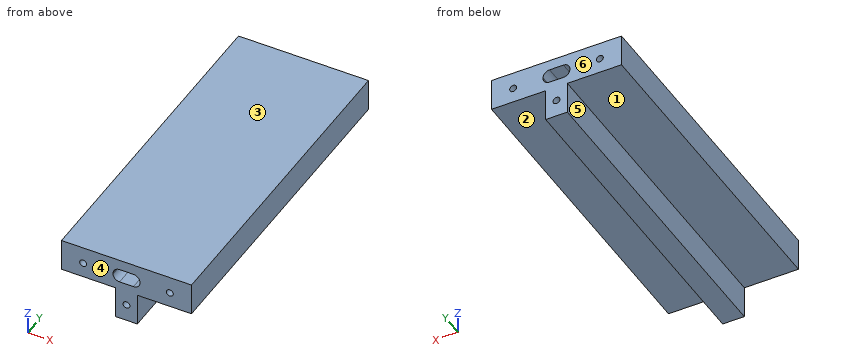
```python
from build123d import *

# Parameters (mm, degrees)
BOSS_EXTRUDE1_DEPTH        = 37.5
SKETCH2_W                  = 6.2
SKETCH2_H                  = 3.2
CUT_EXTRUDE1_DEPTH         = 6.2
FILLET1_R                  = 1.5
M2_TAPPED_HOLE1_AT_2_COUNT = 2
M2_TAPPED_HOLE1_AT_2_PITCH = 12.206555616
M2_TAPPED_HOLE1_AT_3_COUNT = 2
M2_TAPPED_HOLE1_AT_3_PITCH = 20
FILLET1_OF_MIRROR1_R       = 1.5


with BuildPart() as part:
    # Sketch1 → Boss-Extrude1 (new body, symmetric)
    with BuildSketch(Plane(origin=(0, 0, 0), x_dir=(1, 0, 0), z_dir=(0, 1, 0))):
        Polygon((-15, 0), (15, 0), (15, 7.5), (2.5, 7.5), (2.5, 15), (-2.5, 15), (-2.5, 7.5), (-15, 7.5), align=None)
    extrude(amount=BOSS_EXTRUDE1_DEPTH, both=True)

    # Sketch2 → Cut-Extrude1 (cut)
    with BuildSketch(Plane.XZ.offset(37.5)):
        with Locations((0, -4)):
            Rectangle(SKETCH2_W, SKETCH2_H)
    cut_extrude1 = extrude(amount=-CUT_EXTRUDE1_DEPTH, mode=Mode.SUBTRACT)

    # Fillet1
    fillet1_edges = [part.edges().sort_by_distance(p)[0] for p in [
        (-3.1, -34.4, -5.6),
        (-3.1, -34.4, -2.4),
        (3.1, -34.4, -2.4),
        (3.1, -34.4, -5.6),
    ]]
    fillet(fillet1_edges, radius=FILLET1_R)

    # Sketch6 → M2 Tapped Hole1 (revolve, cut)
    with BuildSketch(Plane(origin=(-10, -37.5, -4), x_dir=(0, 0, -1), z_dir=(1, 0, 0))):
        Polygon((0, 0), (0, 5.680688495), (0.8, 5.2), (0.8, 0), align=None)
    m2_tapped_hole1 = revolve(axis=Axis((-10, -43.85, -4), (0, 1, 0)), mode=Mode.SUBTRACT)

    # M2 Tapped Hole1 at 2: M2 Tapped Hole1 ×2
    with Locations(*[Vector(0.819231921, 0, -0.573462344) * (i * M2_TAPPED_HOLE1_AT_2_PITCH) for i in range(1, M2_TAPPED_HOLE1_AT_2_COUNT)]):
        add(m2_tapped_hole1, mode=Mode.SUBTRACT)

    # M2 Tapped Hole1 at 3: M2 Tapped Hole1 ×2
    with Locations(*[(i * M2_TAPPED_HOLE1_AT_3_PITCH, 0, 0) for i in range(1, M2_TAPPED_HOLE1_AT_3_COUNT)]):
        add(m2_tapped_hole1, mode=Mode.SUBTRACT)

    # Mirror1: M2 Tapped Hole1, Cut-Extrude1 across plane
    add(m2_tapped_hole1.mirror(Plane.ZX), mode=Mode.SUBTRACT)
    add(cut_extrude1.mirror(Plane.ZX), mode=Mode.SUBTRACT)

    # Mirror1 copy 1 sketch → Mirror1 copy 1 (revolve, cut)
    with BuildSketch(Plane(origin=(0, 37.5, -11), x_dir=(0, 0, -1), z_dir=(1, 0, 0))):
        Polygon((0, 0), (0, -5.680688495), (0.8, -5.2), (0.8, 0), align=None)
    revolve(axis=Axis((0, 43.85, -11), (0, 1, 0)), mode=Mode.SUBTRACT)

    # Mirror1 copy 2 sketch → Mirror1 copy 2 (revolve, cut)
    with BuildSketch(Plane(origin=(10, 37.5, -4), x_dir=(0, 0, -1), z_dir=(1, 0, 0))):
        Polygon((0, 0), (0, -5.680688495), (0.8, -5.2), (0.8, 0), align=None)
    revolve(axis=Axis((10, 43.85, -4), (0, 1, 0)), mode=Mode.SUBTRACT)

    # Fillet1 of Mirror1
    fillet1_of_mirror1_edges = [part.edges().sort_by_distance(p)[0] for p in [
        (-3.1, 34.4, -5.6),
        (-3.1, 34.4, -2.4),
        (3.1, 34.4, -2.4),
        (3.1, 34.4, -5.6),
    ]]
    fillet(fillet1_of_mirror1_edges, radius=FILLET1_OF_MIRROR1_R)


solid = part.part
```
Geometry check sheet. Reference: the model listing, model coordinates, mm. Face numbers are marked on the shaded views. A direction names the side the tool comes from. Coordinates: 2 decimals unless noted, no trailing zeros. Order: outer loops, then holes, each group sorted by start corner. A loop starts at its lowest first (then second) coordinate and runs counter-clockwise, first axis right, second up.
Q1. Sectioned sample at B-B on x = 6.5. Record the cut outline in (y, z).
Reply:
outline: (-37.5, -7.5) - (37.5, -7.5) - (37.5, 0) - (-37.5, 0) - close
Q2. Sectioned sample at A-A on y = -29.5. Record the cut outline in (x, z).
Reply:
outline: (-15, -7.5) - (-2.5, -7.5) - (-2.5, -15) - (2.5, -15) - (2.5, -7.5) - (15, -7.5) - (15, 0) - (-15, 0) - close
Q3. Sectioned sample at C-C on z = -14. Record the cut outline in (x, y).
Reply:
outline: (-2.5, -37.5) - (2.5, -37.5) - (2.5, 37.5) - (-2.5, 37.5) - close
Q4. Draft check along Y on the marked faces 4, 5 and 6. Enter one of: released by +Y, released by -Y, zero draft, split by the parting line, or undercut.
Reply:
face 4: released by -Y
face 5: zero draft
face 6: released by +Y
Q5. Tool access check on the marked faces 1, 2 and 3. Record the directions out of +Z, -Z, +X, -X, +Y, -Y that give a thin tool (end or side, any length) a straight path to the whole face; none if there is none.
Reply:
face 1: -Z, -X, +Y, -Y
face 2: -Z, +X, +Y, -Y
face 3: +Z, +X, -X, +Y, -Y
Q6. Depth check by flat-ended pin: pin 1 Ø4 at (y, z) = (10, -13) entering from -X; pin 2 Ø3.5 at (x, y) = (1, -34) entering from +Z; pin 3 Ø1 at (x, z) = (0, -11) entering from +Y; pin 4 Ø1.3 at (x, z) = (-10, -4) entering from -Y. Enter the tip coordinate at first touch or a pass-through.
Reply:
pin 1: stops at x = -2.5
pin 2: stops at z = 0
pin 3: stops at y = 32.12
pin 4: stops at y = -32.21
Q7. Thickness scan on probe 1 along Z at (x, y) = (0, 34.95); probe 2 along X at (y, z) = (35.4, -4); probe 3 along X at (y, z) = (35.05, -11). Record the ranges inside material, lowest first.
Reply:
probe 1: z = -15 to -11.8, -10.2 to -5.6, -2.4 to 0
probe 2: x = -15 to -10.8, -9.2 to -3.1, 3.1 to 9.2, 10.8 to 15
probe 3: x = -2.5 to -0.8, 0.8 to 2.5
